Verification items for the finished model (mm, model axes). A direction names the side the tool comes from. Round coordinates to 2 decimals unless told otherwise and drop trailing zeros. Loops run counter-clockwise (first coordinate to the right, second up) from the corner with the lowest first, then second, coordinate; pieces in that order, holes last. Notation, with made-up numbers: (8, -38.75) - (56, -38.75) arc R35 ccw to (56, -3.75) - close; hole circle Ø6 at (14.25, 56). An arc over 180 degrees is marked (long way). Use CSV: the item, a comma, the result in double quotes.
```python
from build123d import *

# Parameters (mm, degrees)
PAD_DEPTH    = 25
SKETCH001_R  = 7
POCKET_DEPTH = 56.001


with BuildPart() as part:
    # Sketch → Pad (new body)
    with BuildSketch(Plane.XY):
        Polygon((-27.014097, -10.624443), (-25.014097, -10.624443), (-25.014097, 53.375557), (26.985903, 53.375557), (26.985903, -10.624443), (28.985903, -10.624443), (28.985903, 55.375557), (-27.014097, 55.375557), align=None)
    extrude(amount=PAD_DEPTH)

    # Sketch001 (on Face6 of Pad) → Pocket (cut, through all)
    with BuildSketch(Plane.YZ.offset(28.985903)):
        with Locations((2.875557, 12.5)):
            Circle(SKETCH001_R)
    extrude(amount=-POCKET_DEPTH, mode=Mode.SUBTRACT)


with BuildPart() as part_1:
    # Body placement: moved
    add(part.part.moved(Location((0, -3, -12.5))))


solid = part_1.part
```
1) Cross-section at C-C, the plane x = -21. Record the cut outline in (y, z), then the cut area to 3 significant figures.
Returned:
outline,"(50.38, -12.5) - (52.38, -12.5) - (52.38, 12.5) - (50.38, 12.5) - close"
area,"50.0 mm²"
2) Thickness scan on probe 1 along X at (y, z) = (12.5, 0.25); probe 2 along Y at (x, z) = (9.5, -8.5). Record the ranges inside material, lowest first. Write a range as [from, to].
Returned:
probe 1,"x = [-27.01, -25.01], [26.99, 28.99]"
probe 2,"y = [50.38, 52.38]"
3) Cross-section at B-B, the plane y = 34.5. Record the cut outline in (x, z).
Returned:
outline,"(-27.01, -12.5) - (-25.01, -12.5) - (-25.01, 12.5) - (-27.01, 12.5) - close; (26.99, -12.5) - (28.99, -12.5) - (28.99, 12.5) - (26.99, 12.5) - close"
4) Cross-section at A-A, the plane z = 0. Record the cut outline in (x, y).
Returned:
outline,"(-27.01, -13.62) - (-25.01, -13.62) - (-25.01, -7.12) - (-27.01, -7.12) - close; (-27.01, 6.88) - (-25.01, 6.88) - (-25.01, 50.38) - (26.99, 50.38) - (26.99, 6.88) - (28.99, 6.88) - (28.99, 52.38) - (-27.01, 52.38) - close; (26.99, -13.62) - (28.99, -13.62) - (28.99, -7.12) - (26.99, -7.12) - close"
5) Access from +Z, -Z, +X, -X, +Y, -Y to the whole of each face (thin tool, end or side, straight path). Record for faces 4 (the face through (-25.014, 18, 0)), 5 (the face through (28, -13.624, 0)).
Returned:
face 4,"+Z, -Z, -Y"
face 5,"+Z, -Z, +X, -X, -Y"
6) Gauge pin test, flat end, axial feed: pin 1 Ø2 at (x, z) = (-10.5, -1.5) entering from -Y. Record the tip position at first contact, or that the pin passes through.
Returned:
pin 1,"stops at y = 50.38"
7) Mould release check, pull along X, two halves, no side actions. Record for faces 1 (the face through (-27.014, 20, 0)), 2 (the face through (26.986, 19, 0)), 3 (the face through (1, 51, -12.5)): +X half, -X half, draft (parallel to the pull), parting line (faces both ways), or undercut.
Returned:
face 1,"-X half"
face 2,"undercut"
face 3,"draft"
